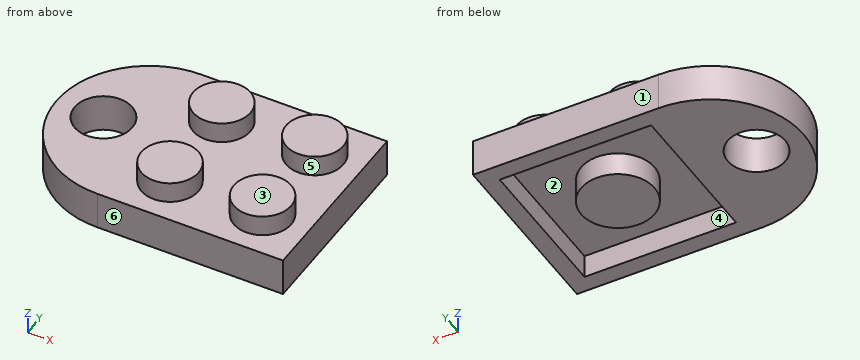
from build123d import *

# Parameters (mm, degrees)
F0_W     = 15.82
F0_H     = 15.82
F1_DEPTH = 3.25
F2_R     = 2.44
F3_DEPTH = 1.8
F4_W     = 12.9
F4_H     = 12.9
F4_R     = 3.125
F5_DEPTH = 2.01
F6_R     = 2.45
F7_DEPTH = 25


with BuildPart() as f1:
    # F0 (on Top) → F1 (new body)
    with BuildSketch(Plane.XY):
        with Locations((1.526456, -1.522328)):
            Rectangle(F0_W, F0_H)
        with BuildLine():
            ThreePointArc((-6.383544, 6.387672), (-14.293544, -1.522328), (-6.383544, -9.432328))
            Line((-6.383544, -9.432328), (-6.383544, 6.387672))
        make_face()
    extrude(amount=F1_DEPTH)

    # F2 (on face) → F3 (join)
    with BuildSketch(Plane.XY.offset(3.25)):
        with Locations((-2.423831, 2.437297)):
            Circle(F2_R)
        with Locations((5.484728, 2.457458)):
            Circle(F2_R)
        with Locations((5.483022, -5.48487)):
            Circle(F2_R)
        with Locations((-2.401933, -5.481959)):
            Circle(F2_R)
    extrude(amount=F3_DEPTH)

    # F4 (on face) → F5 (cut)
    with BuildSketch(Plane.XY):
        with Locations((1.526456, -1.522328)):
            Rectangle(F4_W, F4_H)
        with Locations((1.526456, -1.522328)):
            Circle(F4_R, mode=Mode.SUBTRACT)
    extrude(amount=F5_DEPTH, mode=Mode.SUBTRACT)

    # F6 (on face) → F7 (cut)
    with BuildSketch(Plane.XY.offset(3.25)):
        with Locations((-10.308685, -1.488805)):
            Circle(F6_R)
    extrude(amount=-F7_DEPTH, mode=Mode.SUBTRACT)


solid = f1.part
Input: part model. Units: mm. Frame: model coordinates. Face numbers are marked on the shaded views. A direction names the side the tool comes from. Give positions to 0.01 mm unless a question says otherwise; leave off trailing zeros. Order: outer loops, then holes, each group sorted by start corner. A loop starts at its lowest first (then second) coordinate and runs counter-clockwise, first axis right, second up. Notation, with made-up numbers: M 26.5,41 L 79.5,41 A7 ccw 79.5,45 Z; hole C -5.5,27 d6. An arc over 180 degrees is marked long. Answer as a JSON object with one key per item and string values.
1. Cut plane D-D, the plane z = 3.7. Output: boundary loops of the cut face in (x, y), and give its area (3 significant figures).
Result sheet:
{"outline": "C -2.42,2.44 d4.88; C -2.4,-5.48 d4.88; C 5.48,-5.48 d4.88; C 5.48,2.46 d4.88", "area": "74.8 mm²"}
2. Ray query, line 1 (Y direction, x = -4.5, z = 0.4); line 2 (Z direction, x = 6.5, y = -1.5); line 3 (Z direction, x = -2.25, y = -5.75). Return the intervals inside material, ascending. Write a range as [from, to].
Result sheet:
{"line 1": "[-9.43, -7.97], [4.93, 6.39]", "line 2": "[2.01, 3.25]", "line 3": "[2.01, 5.05]"}
3. Cut plane B-B, the plane y = 0.5. Output: boundary loops of the cut face in (x, z).
Result sheet:
{"outline": "M -14.03,0 L -11.74,0 L -11.74,3.25 L -14.03,3.25 Z; M -8.88,0 L -4.92,0 L -4.92,2.01 L -0.86,2.01 L -0.86,0 L 3.91,0 L 3.91,2.01 L 7.98,2.01 L 7.98,0 L 9.44,0 L 9.44,3.25 L 6.94,3.25 L 6.94,5.05 L 4.03,5.05 L 4.03,3.25 L -0.94,3.25 L -0.94,5.05 L -3.91,5.05 L -3.91,3.25 L -8.88,3.25 Z"}
4. Reachability of the marked faces 4, 5 and 6 from +Z, -Z, +X, -X, +Y, -Y: full face, straight path, thin tool, end or side. Return the list, or none.
Result sheet:
{"face 4": "-Z", "face 5": "+Z", "face 6": "+Z, -Z, +X, -X, -Y"}
5. Cut plane C-C, the plane x = -11. Output: boundary loops of the cut face in (y, z).
Result sheet:
{"outline": "M -7.95,0 L -3.84,0 L -3.84,3.25 L -7.95,3.25 Z; M 0.86,0 L 4.9,0 L 4.9,3.25 L 0.86,3.25 Z"}
6. Pull-direction query (Y, two-part tool) for the marked faces 1, 2 and 3; classes: +Y half, -Y half, draft (parallel to the pull), parting line (faces both ways), or undercut.
Result sheet:
{"face 1": "+Y half", "face 2": "undercut", "face 3": "draft"}
7. Cut plane A-A, the plane z = 1.6. Output: boundary loops of the cut face in (x, y) (3 decimals).
Result sheet:
{"outline": "M -6.384,-9.432 L 9.436,-9.432 L 9.436,6.388 L -6.384,6.388 A7.91 ccw Z; C 1.526,-1.522 d6.25; hole C -10.309,-1.489 d4.9; hole M -4.924,-7.972 L 7.976,-7.972 L 7.976,4.928 L -4.924,4.928 Z"}
8. First-contact query: P1, Ø1, axis at y = -4.5, z = 1.5, coming from the -X side; P2, Ø1, axis at x = 4.5, z = 4, coming from the +Y side; P3, Ø1, axis at x = -11, y = 2, coming from the +Z side. Flat tips, straight axial feed; report the tip coordinate or a pass-through.
Result sheet:
{"P1": "x = -13.9", "P2": "y = 4.85", "P3": "z = 3.25"}
